Verification items for the finished model (mm, model axes). Face numbers are marked on the shaded views. A direction names the side the tool comes from. Round coordinates to 2 decimals unless told otherwise and drop trailing zeros. Order: outer loops, then holes, each group sorted by start corner. A loop starts at its lowest first (then second) coordinate and runs counter-clockwise, first axis right, second up. Notation, with made-up numbers: M -38,22 L 1,22 A34 ccw 1,58 Z; hole C 42,63 d3. An arc over 180 degrees is marked long. Use one line per item in the form item = value. Start each with the question number.
Item 1: Thickness scan on probe 1 along Z at (x, y) = (-0.5, 1.75); probe 2 along Y at (x, z) = (0, 3.75); probe 3 along Y at (x, z) = (7, 11). Record the ranges inside material, lowest first. Write a range as [from, to].
Item 2: Cross-section at D-D on x = -7. Enter the section's corners in (y, z) (3 decimals).
Item 3: Release check for a two-part mould opening along X. For the marked faces 1, 2 and 3 record: +X half, -X half, draft (parallel to the pull), parting line (faces both ways), or undercut.
Item 4: Go/stop test with flat-tipped pins: pin 1 Ø3 at (x, y) = (13, 10) entering from -Z; pin 2 Ø1.5 at (y, z) = (8.5, -10.5) entering from +X; pin 3 Ø4 at (x, y) = (0.5, 1.5) entering from +Z; pin 4 Ø1.5 at (x, z) = (-15.5, 9) entering from +Y. Record where each tip stops, or that it passes through.
Item 5: Cross-section at B-B on z = 0. Enter the section's corners in (x, y).
Item 6: Cross-section at A-A on x = 0. Enter the section's corners in (y, z), then the cut area to 3 significant figures.
Item 7: Tool access check on the marked faces 4 and 5. Record the directions out of +Z, -Z, +X, -X, +Y, -Y that give a thin tool (end or side, any length) a straight path to the whole face; none if there is none.
Item 8: Cross-section at C-C on y = 5. Enter the section's corners in (x, z).
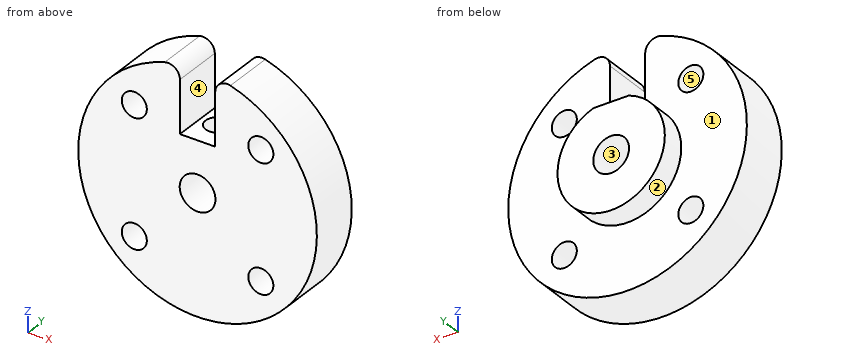
from build123d import *

# Parameters (mm, degrees)
SKETCH1_R                  = 9
SKETCH1_R_2                = 3
BOSS_EXTRUDE1_DEPTH        = 12.5
SKETCH5_W                  = 2.1
SKETCH5_H                  = 9
CUT_EXTRUDE1_START         = 9
SKETCH6_W                  = 18
SKETCH6_H                  = 12.5
CUT_EXTRUDE1_DEPTH         = 0.5
BOSS_EXTRUDE2_DEPTH        = 8.5
FILLET1_R                  = 2
F_4_2_4_2_DIAMETER_HOLE2_D = 4.2


with BuildPart() as part:
    # Sketch1 → Boss-Extrude1 (new body)
    with BuildSketch(Plane(origin=(0, 0, 0), x_dir=(1, 0, 0), z_dir=(0, 1, 0))):
        with Locations(Location((0, 0, 0), (0, 0, 270))):
            Circle(SKETCH1_R)
        with Locations(Location((0, 0, 0), (0, 0, 270))):
            Circle(SKETCH1_R_2, mode=Mode.SUBTRACT)
    extrude(amount=BOSS_EXTRUDE1_DEPTH)

    # Sketch5 → Ø4.2 (4.2) Diameter Hole1 (revolve, cut)
    with BuildSketch(Plane(origin=(0, 5, 0), x_dir=(0, 1, 0), z_dir=(1, 0, 0))):
        with Locations((1.05, 4.5)):
            Rectangle(SKETCH5_W, SKETCH5_H)
    revolve(axis=Axis((0, 5, -6.35), (0, 0, 1)), mode=Mode.SUBTRACT)

    # Sketch6 → Cut-Extrude1 (cut)
    with BuildSketch(Plane.XY.offset(CUT_EXTRUDE1_START)):
        with Locations((0, 6.25)):
            Rectangle(SKETCH6_W, SKETCH6_H)
    extrude(amount=-CUT_EXTRUDE1_DEPTH, mode=Mode.SUBTRACT)

    # Sketch7 → Boss-Extrude2 (add)
    with BuildSketch(Plane.XZ):
        with BuildLine():
            Line((-2.958039892, 8.5), (-2.958039892, 19.780040445))
            ThreePointArc((-2.958039892, 19.780040445), (0, -20), (2.958039892, 19.780040445))
            Line((2.958039892, 19.780040445), (2.958039892, 8.5))
            ThreePointArc((2.958039892, 8.5), (0, -9), (-2.958039892, 8.5))
        make_face()
    extrude(amount=-BOSS_EXTRUDE2_DEPTH)

    # Fillet1
    fillet1_edges = [part.edges().sort_by_distance(p)[0] for p in [
        (-2.958039892, 4.25, 19.780040445),
        (2.958039892, 4.25, 19.780040445),
    ]]
    fillet(fillet1_edges, radius=FILLET1_R)

    # Ø4.2 (4.2) Diameter Hole2 (through all)
    with Locations(Plane(origin=(0, 0, 0), x_dir=(-1, 0, 0), z_dir=(0, -1, 0))):
        with Locations((10.606601718, -10.606601718), (-10.606601718, -10.606601718), (-10.606601718, 10.606601718), (10.606601718, 10.606601718)):
            Hole(F_4_2_4_2_DIAMETER_HOLE2_D / 2)


solid = part.part
Output values:
q1.probe_1 = [-19.99, -2.96], [2.96, 8.5]
q1.probe_2 = [0, 2.9], [7.1, 12.5]
q1.probe_3 = [0, 8.5]
q2.outline = M 0,-18.735 L 8.5,-18.735 L 8.5,-5.657 L 12.5,-5.657 L 12.5,5.657 L 8.5,5.657 L 8.5,18.735 L 0,18.735 Z
q3.face_1 = draft
q3.face_2 = parting line
q3.face_3 = undercut
q4.pin_1 = through
q4.pin_2 = 17.46
q4.pin_3 = 8.5
q4.pin_4 = 8.5
q5.outline = M -20,0 L -3,0 L -3,12.5 L -9,12.5 L -9,8.5 L -20,8.5 Z; M 3,0 L 20,0 L 20,8.5 L 9,8.5 L 9,12.5 L 3,12.5 Z
q6.outline = M 0,-20 L 8.5,-20 L 8.5,-9 L 12.5,-9 L 12.5,-3 L 0,-3 Z; M 0,3 L 2.9,3 L 2.9,8.5 L 0,8.5 Z; M 7.1,3 L 12.5,3 L 12.5,8.5 L 7.1,8.5 Z
q6.area = 214 mm2
q7.face_4 = +Z, +Y, -Y
q7.face_5 = +Y, -Y
q8.outline = M -5.51,19.23 A20 ccw long 5.51,19.23 A2 ccw 2.96,17.3 L 2.96,8.5 L 2.1,8.5 L 2.1,2.14 A3 cw long -2.1,2.14 L -2.1,8.5 L -2.96,8.5 L -2.96,17.3 A2 ccw Z; hole C -10.61,-10.61 d4.2; hole C -10.61,10.61 d4.2; hole C 10.61,-10.61 d4.2; hole C 10.61,10.61 d4.2
